from build123d import *

# Parameters (mm, degrees)
F0_R     = 3.1
F1_DEPTH = 3
F2_W     = 26
F2_H     = 20
F3_DEPTH = 10
F4_SIZE  = 2
F6_DEPTH = 2
F8_DEPTH = 2


with BuildPart() as f1:
    # F0 (on Top) → F1 (new body)
    with BuildSketch(Plane.XY):
        Polygon((-13, -10), (13, -10), (28, -10), (28, 10), (13, 10), (-13, 10), align=None)
        Circle(F0_R, mode=Mode.SUBTRACT)
        with Locations((20.5, 0)):
            Circle(F0_R, mode=Mode.SUBTRACT)
    extrude(amount=F1_DEPTH)

    # F2 (on face) → F3 (join)
    with BuildSketch(Plane.XY.offset(3)):
        Rectangle(F2_W, F2_H)
        with BuildLine():
            ThreePointArc((-10, 2.757359), (-10, 7), (-5.757359, 7))
            Line((-5.757359, 7), (5.757359, 7))
            ThreePointArc((5.757359, 7), (10, 7), (10, 2.757359))
            Line((10, 2.757359), (10, -2.757359))
            ThreePointArc((10, -2.757359), (10, -7), (5.757359, -7))
            Line((5.757359, -7), (-5.757359, -7))
            ThreePointArc((-5.757359, -7), (-10, -7), (-10, -2.757359))
            Line((-10, -2.757359), (-10, 2.757359))
        make_face(mode=Mode.SUBTRACT)
    extrude(amount=F3_DEPTH)

    # F4
    f4_edges = [f1.edges().sort_by_distance(p)[0] for p in [
        (0, -10, 13),
        (13, 0, 13),
        (0, 10, 13),
        (-13, 0, 13),
    ]]
    chamfer(f4_edges, length=F4_SIZE)

    # F5 (on face) → F6 (join)
    with BuildSketch(Plane.XZ.offset(10)):
        Polygon((28, 3), (13, 11), (13, 3), align=None)
    extrude(amount=-F6_DEPTH)

    # F7 (on face) → F8 (join)
    with BuildSketch(Plane(origin=(0, 10, 0), x_dir=(-1, 0, 0), z_dir=(0, 1, 0))):
        Polygon((-13, 3), (-13, 11), (-28, 3), align=None)
    extrude(amount=-F8_DEPTH)


solid = f1.part
Verification items for the finished model (mm, model axes). A direction names the side the tool comes from. Coordinates: 2 decimals unless noted, no trailing zeros. Write each loop counter-clockwise with the first axis right and the second up, starting at its lowest first coordinate (ties: lowest second). Pieces come first, ordered by that corner, then holes. Notation, with made-up numbers: M -31.75,32.5 L -17.75,32.5 A7 cw -17.75,40.5 Z; hole C -21,16 d8. An arc over 180 degrees is marked long. Use a Markdown table: item, result.
Q1. Draft check along Y on faces 1 (the face through (0, -7, 8)), 2 (the face through (-13, 0, 5)), 3 (the face through (3, -10, 6)). Enter one of: +Y half, -Y half, draft (parallel to the pull), parting line (faces both ways), or undercut.
Reply:
| item | result |
|---|---|
| face 1 | undercut |
| face 2 | draft |
| face 3 | -Y half |
Q2. Thickness scan on line 1 (Y direction, x = 0, z = 1.9); line 2 (X direction, y = 5, z = 4); line 3 (Y direction, x = 3, z = 4.5). Record the ranges inside material, lowest first.
Reply:
| item | result |
|---|---|
| line 1 | y = -10 to -3.1, 3.1 to 10 |
| line 2 | x = -13 to -10.88, 10.88 to 13 |
| line 3 | y = -10 to -7, 7 to 10 |
Q3. Sectioned sample at C-C, the plane z = 1.75. Record the boundary of the cut face in (x, y).
Reply:
| item | result |
|---|---|
| outline | M -13,-10 L 28,-10 L 28,10 L -13,10 Z; hole C 0,0 d6.2; hole C 20.5,0 d6.2 |
Q4. Sectioned sample at D-D, the plane z = 9. Record the boundary of the cut face in (x, y).
Reply:
| item | result |
|---|---|
| outline | M -13,-10 L 16.75,-10 L 16.75,-8 L 13,-8 L 13,8 L 16.75,8 L 16.75,10 L -13,10 Z; hole M -10,-2.76 A3 ccw -5.76,-7 L 5.76,-7 A3 ccw 10,-2.76 L 10,2.76 A3 ccw 5.76,7 L -5.76,7 A3 ccw -10,2.76 Z |
Q5. Sectioned sample at B-B, the plane x = 0. Record the boundary of the cut face in (y, z), plus the area to 3 significant figures.
Reply:
| item | result |
|---|---|
| outline | M -10,0 L -3.1,0 L -3.1,3 L -7,3 L -7,13 L -8,13 L -10,11 Z; M 3.1,0 L 10,0 L 10,11 L 8,13 L 7,13 L 7,3 L 3.1,3 Z |
| area | 97.4 mm² |
Q6. Set-up check for faces 4 (the face through (13, 0, 7)), 5 (the face through (-10, -7, 8)), 6 (the face through (0, 9, 12)): record each of +Z, -Z, +X, -X, +Y, -Y from which the full face is reachable in a straight line by a thin tool's end or side.
Reply:
| item | result |
|---|---|
| face 4 | +Z, +X |
| face 5 | +Z |
| face 6 | +Z, +X, -X, +Y |
Q7. Go/stop test with flat-tipped pins: P1, Ø5, axis at x = 20.5, y = 0, coming from the -Z side; P2, Ø8, axis at x = 1, y = -0.5, coming from the +Z side. Record where each tip stops, or that it passes through.
Reply:
| item | result |
|---|---|
| P1 | passes through |
| P2 | stops at z = 3 |
Q8. Sectioned sample at A-A, the plane y = 0. Record the boundary of the cut face in (x, z).
Reply:
| item | result |
|---|---|
| outline | M -13,0 L -3.1,0 L -3.1,3 L -10,3 L -10,13 L -11,13 L -13,11 Z; M 3.1,0 L 17.4,0 L 17.4,3 L 13,3 L 13,11 L 11,13 L 10,13 L 10,3 L 3.1,3 Z; M 23.6,0 L 28,0 L 28,3 L 23.6,3 Z |
